Read the model definition and answer for the solid it produces. Units are mm, in the model's axes. A direction names the side the tool comes from. Coordinates: 2 decimals unless noted, no trailing zeros. Write each loop counter-clockwise with the first axis right and the second up, starting at its lowest first coordinate (ties: lowest second). Pieces come first, ordered by that corner, then holes. Notation, with made-up numbers: (74.25, -12) -> (129.25, -12) arc R31 ccw to (129.25, 16) -> close; hole circle Ø10 at (25, 40.5). An arc over 180 degrees is marked (long way). Answer in a Markdown table with one row per item. Add a question column.
Item 1: Section A-A on y = 7 is taken. Write down the section's boundary in (x, z) (3 decimals), then the cut area to 3 significant figures.
Item 2: Given pin 1 Ø8 at (y, z) = (13.5, 13) entering from -X; pin 2 Ø1 at (x, z) = (9, 17) entering from -Y (3 decimals); pin 3 Ø6 at (y, z) = (4.5, -3) entering from -X, each flat-ended and moving along its own axis, determine where each tip first touches the part or whether it passes through.
Item 3: For a pull along Z with two mould halves and no side action, classify faces 1 (the face through (0, 0, 21)), 2 (the face through (25.17, 8.37, -25.03)), 3 (the face through (0, 8, -20.32)), 4 (the face through (0, 8, 25.4)) as +Z half, -Z half, draft (parallel to the pull), parting line (faces both ways), or undercut.
Item 4: Straight lines are drawn through the part: line 1 (Z direction, x = 9.5, y = 4.25); line 2 (Y direction, x = -17, z = -11) (3 decimals); line 3 (X direction, y = 13.5, z = -16.5). For each, find the intervals that lie inside material, in ascending order. Write a range as from..to.
Item 5: Section B-B on x = -1.5 is taken. Write down the section's boundary in (y, z) (3 decimals), then the cut area to 3 significant figures.
Item 6: Which of the six approach directions +Z, -Z, +X, -X, +Y, -Y give full straight-line access (tool end or side, diameter ignored) to faces 5 (the face through (0, 15.875, 0)), 6 (the face through (31.75, 8.14, -0.35))?
```python
from build123d import *

# Parameters (mm, degrees)
SKETCH1_W           = 50.8
SKETCH1_H           = 50.8
BOSS_EXTRUDE1_DEPTH = 19.05
SKETCH2_W           = 45.72
SKETCH2_H           = 40.64
CUT_EXTRUDE1_DEPTH  = 15.875
FILLET1_R           = 2.54


with BuildPart() as part:
    # Sketch1 → Boss-Extrude1 (new body)
    with BuildSketch(Plane(origin=(0, 0, 0), x_dir=(1, 0, 0), z_dir=(0, 1, 0))):
        with BuildLine():
            ThreePointArc((-25.4, -25.4), (-31.75, 0), (-25.4, 25.4))
            Line((-25.4, 25.4), (-25.4, -25.4))
        make_face()
        with BuildLine():
            ThreePointArc((25.4, 25.4), (31.75, 0), (25.4, -25.4))
            Line((25.4, -25.4), (25.4, 25.4))
        make_face()
        Rectangle(SKETCH1_W, SKETCH1_H)
    extrude(amount=BOSS_EXTRUDE1_DEPTH)

    # Sketch2 → Cut-Extrude1 (cut)
    with BuildSketch(Plane.XZ):
        Rectangle(SKETCH2_W, SKETCH2_H)
    extrude(amount=-CUT_EXTRUDE1_DEPTH, mode=Mode.SUBTRACT)

    # Fillet1
    fillet1_edges = [part.edges().sort_by_distance(p)[0] for p in [
        (31.75, 19.05, 0),
        (0, 19.05, -25.4),
        (-31.75, 19.05, 0),
        (0, 19.05, 25.4),
        (-25.4, 9.525, -25.4),
        (25.4, 9.525, -25.4),
        (25.4, 9.525, 25.4),
        (-25.4, 9.525, 25.4),
    ]]
    fillet(fillet1_edges, radius=FILLET1_R)


solid = part.part
```
Results below:
| question | item | result |
|---|---|---|
| 1 | outline | (-26.126, -23.989) arc R2.54 ccw to (-23.851, -25.4) -> (23.851, -25.4) arc R2.54 ccw to (26.126, -23.989) arc R53.975 ccw to (26.126, 23.989) arc R2.54 ccw to (23.851, 25.4) -> (-23.851, 25.4) arc R2.54 ccw to (-26.126, 23.989) arc R53.975 ccw to start; hole (-22.86, -20.32) -> (22.86, -20.32) -> (22.86, 20.32) -> (-22.86, 20.32) -> close |
| 1 | area | 1,160 mm2 |
| 2 | pin 1 | stops at x = -30.99 |
| 2 | pin 2 | stops at y = 15.875 |
| 2 | pin 3 | stops at x = -31.75 |
| 3 | face 1 | draft |
| 3 | face 2 | -Z half |
| 3 | face 3 | undercut |
| 3 | face 4 | +Z half |
| 4 | line 1 | z = -25.4..-20.32, 20.32..25.4 |
| 4 | line 2 | y = 15.875..19.05 |
| 4 | line 3 | x = -29.17..-22.86, 22.86..29.17 |
| 5 | outline | (0, -25.4) -> (16.51, -25.4) arc R2.54 ccw to (19.05, -22.86) -> (19.05, 22.86) arc R2.54 ccw to (16.51, 25.4) -> (0, 25.4) -> (0, 20.32) -> (15.875, 20.32) -> (15.875, -20.32) -> (0, -20.32) -> close |
| 5 | area | 320 mm2 |
| 6 | face 5 | -Y |
| 6 | face 6 | +X, +Y, -Y |
